Design review of the part built by this model. Coordinates are the model's own, in mm. A direction names the side the tool comes from. Coordinates: 2 decimals unless noted, no trailing zeros. Loops run counter-clockwise (first coordinate to the right, second up) from the corner with the lowest first, then second, coordinate; pieces in that order, holes last.
Autodesk Inventor part; units mm, degrees
ref_plane "YZ Plane" through (0, 0, 0) normal (1, 0, 0) x (0, 1, 0)
ref_plane "XZ Plane" through (0, 0, 0) normal (0, 1, 0) x (-1, 0, 0)
ref_plane "XY Plane" through (0, 0, 0) normal (0, 0, 1) x (1, 0, 0)
sketch "Sketch1" plane through (0, 0, 0) normal (0, 0, 1) x (1, 0, 0)
  line L0 (0, 0) -> (60, 0)
  line L1 (60, 0) -> (60, 40)
  line L2 (60, 40) -> (0, 40)
  line L3 (0, 40) -> (0, 0)
  circle A0 centre (60, 20) radius 15
  circle A1 centre (47.5, 20) radius 1.4
  circle A2 centre (60, 7.5) radius 1.4
  circle A3 centre (72.5, 20) radius 1.4
  circle A4 centre (60, 32.5) radius 1.4
  point P0 (60, 5)
  point P1 (60, 35)
  dimension "d0" = 60
  dimension "d1" = 40
  dimension "d2" = 30
  dimension "d3" = 2.8
  dimension "d4" = 12.5
  dimension "d7" = 360
extrude "Extrusion1" add sketch "Sketch1" along normal blind 7 contours L3 L2 L1 A0 L0 | A0 L1 A4 A2 | L1 A2 A4 A0
sketch "Sketch2" plane through (0, 0, 7) normal (0, 0, 1) x (1, 0, 0)
  line L0 (13, 36) -> (36, 36)
  line L1 (36, 36) -> (36, 4)
  line L2 (36, 4) -> (13, 4)
  line L3 (13, 4) -> (13, 36)
  line L4 (0, 40) -> (0, 0)
  circle A0 centre (13, 36) radius 1.4
  line L5 (0, 20) -> (36, 20)
  circle A1 centre (13, 4) radius 1.4
  line L6 (24.5, 36) -> (24.5, 4)
  circle A2 centre (36, 36) radius 1.4
  circle A3 centre (36, 4) radius 1.4
  dimension "d11" = 23
  dimension "d12" = 32
  dimension "d13" = 2.8
  dimension "d22" = 13
extrude "Extrusion2" cut sketch "Sketch2" against normal through all contours L3 A0 L0 | L0 A0 L3 | A2 L1 L0 | L0 L1 A2 | A1 L2 L3 | L3 L2 A1 | A3 L2 L1 | L1 L2 A3
sketch "Sketch3" plane through (0, 0, 7) normal (0, 0, 1) x (1, 0, 0)
  line L0 (5, 36) -> (28, 36)
  line L1 (28, 36) -> (28, 4)
  line L2 (28, 4) -> (5, 4)
  line L3 (5, 4) -> (5, 36)
  line L4 (0, 40) -> (0, 0)
  circle A0 centre (36, 36) radius 1.4
  circle A1 centre (5, 36) radius 1.4
  line L5 (0, 20) -> (28, 20)
  circle A2 centre (5, 4) radius 1.4
  line L6 (16.5, 36) -> (16.5, 4)
  circle A3 centre (28, 36) radius 1.4
  circle A4 centre (28, 4) radius 1.4
  point P0 (5, 20)
  dimension "d16" = 23
  dimension "d17" = 32
  dimension "d18" = 8
  dimension "d19" = 2.8
extrude "Extrusion3" cut sketch "Sketch3" against normal through all contours L3 A1 L0 | L0 A1 L3 | A3 L1 L0 | L0 L1 A3 | A2 L2 L3 | L3 L2 A2 | A4 L2 L1 | L1 L2 A4
properties part number "üst döner tablo1"
Q1. Machinability: for faces 4 (the flat face through (60, 2, 3)), 5 (the cylindrical face through (48.79, 20.54, 3.45)), which of the approach directions +Z, -Z, +X, -X, +Y, -Y give a long, thin tool a straight path to every point of the face, cutting with its end or side? Answer none if there is none.
Q2. The part is to be moulded in two halves that separate along X. For faces 1 (the flat face through (37, 20, 0)), 2 (the flat face through (60, 37, 3)), 3 (the cylindrical face through (12.82, 37.39, 3.55)), say which applies: pulls with the +X half, pulls with the -X half, needs draft (parallel to the pull), parting line crosses it, or undercut.
Q3. Clearance check with flat-ended pins moving along their axes: pin 1 Ø2 at (y, z) = (24.5, 3) entering from -X; pin 2 Ø1.5 at (y, z) = (37.5, 4.5) entering from +X. State where each tip first meets the part, or that it passes through.
Q4. Take a section at C-C, the plane y = 20. Write out the cut boundary in (x, z).
Q5. Take a section at D-D, the plane x = 13. Write out the cut boundary in (y, z), then the cut area to 3 significant figures.
Q6. Take a section at A-A, the plane x = 47.5. Write out the cut boundary in (y, z), then the cut area to 3 significant figures.
Q7. Take a section at B-B, the plane z = 2.75. Give the number of separate pieces and of enclosed holes in the cut face, then the cut area to 3 significant figures.
Q8. For line 1 (X direction, y = 36, z = 2); line 2 (Y direction, x = 28, z = 4.75); line 3 (Y direction, x = 13.5, z = 3.25), list the stretches that pass through material, from the lowest coordinate up.
Entries:
1. face 4: +Z, -Z, +X, -Y
1. face 5: +Z, -Z
2. face 1: needs draft
2. face 2: pulls with the +X half
2. face 3: undercut
3. pin 1: stops at x = 0
3. pin 2: stops at x = 60
4. outline: (0, 0) - (46.1, 0) - (46.1, 7) - (0, 7) - close; (48.9, 0) - (71.1, 0) - (71.1, 7) - (48.9, 7) - close; (73.9, 0) - (75, 0) - (75, 7) - (73.9, 7) - close
5. outline: (0, 0) - (2.6, 0) - (2.6, 7) - (0, 7) - close; (5.4, 0) - (34.6, 0) - (34.6, 7) - (5.4, 7) - close; (37.4, 0) - (40, 0) - (40, 7) - (37.4, 7) - close
5. area: 241 mm2
6. outline: (0, 0) - (18.6, 0) - (18.6, 7) - (0, 7) - close; (21.4, 0) - (40, 0) - (40, 7) - (21.4, 7) - close
6. area: 260 mm2
7. separate pieces: 1
7. enclosed holes: 12
7. area: 2,680 mm2
8. line 1: x = 0 to 3.6, 6.4 to 11.6, 14.4 to 26.6, 29.4 to 34.6, 37.4 to 60
8. line 2: y = 0 to 2.6, 5.4 to 34.6, 37.4 to 40
8. line 3: y = 0 to 2.69, 5.31 to 34.69, 37.31 to 40
